Source: CAD feature listing. Evaluate the final solid. Frame: model axes, mm. A direction names the side the tool comes from. Give positions to 0.01 mm unless a question says otherwise; leave off trailing zeros. Order: outer loops, then holes, each group sorted by start corner. A loop starts at its lowest first (then second) coordinate and runs counter-clockwise, first axis right, second up.
```python
from build123d import *

# Parameters (mm, degrees)
SKETCH1_W           = 25.4
SKETCH1_H           = 23.622
BOSS_EXTRUDE1_DEPTH = 5.842
SKETCH2_R           = 3.175
CUT_EXTRUDE1_DEPTH  = 36.175102672
SKETCH3_R           = 7.14375
CUT_EXTRUDE2_DEPTH  = 4.9022
CUT_EXTRUDE3_DEPTH  = 36.175102672
CUT_EXTRUDE4_DEPTH  = 36.175102672
SKETCH6_W           = 7
SKETCH6_H           = 5
CUT_EXTRUDE5_DEPTH  = 36.175102828
SKETCH8_R           = 1.1303
CUT_EXTRUDE6_DEPTH  = 6.35


with BuildPart() as part:
    # Sketch1 → Boss-Extrude1 (new body)
    with BuildSketch(Plane(origin=(0, 0, 0), x_dir=(1, 0, 0), z_dir=(0, 1, 0))):
        with Locations((12.7, 11.811)):
            Rectangle(SKETCH1_W, SKETCH1_H)
    extrude(amount=BOSS_EXTRUDE1_DEPTH)

    # Sketch2 → Cut-Extrude1 (cut, through all)
    with BuildSketch(Plane(origin=(0, 5.842, 0), x_dir=(1, 0, 0), z_dir=(0, 1, 0))):
        with Locations(Location((12.7, 15.24, 0), (0, 0, 270))):
            Circle(SKETCH2_R)
    extrude(amount=-CUT_EXTRUDE1_DEPTH, mode=Mode.SUBTRACT)

    # Sketch3 → Cut-Extrude2 (cut)
    with BuildSketch(Plane(origin=(0, 5.842, 0), x_dir=(1, 0, 0), z_dir=(0, 1, 0))):
        with Locations(Location((12.7, 15.24, 0), (0, 0, 270))):
            Circle(SKETCH3_R)
    extrude(amount=-CUT_EXTRUDE2_DEPTH, mode=Mode.SUBTRACT)

    # Sketch4 → Cut-Extrude3 (cut, through all)
    with BuildSketch(Plane(origin=(0, 5.842, 0), x_dir=(1, 0, 0), z_dir=(0, 1, 0))):
        with BuildLine():
            ThreePointArc((4.318, 15.24), (6.77303096, 21.16696904), (12.7, 23.622))
            Line((12.7, 23.622), (0, 23.622))
            Line((0, 23.622), (0, 3.302))
            ThreePointArc((0, 3.302), (3.053287081, 4.566712919), (4.318, 7.62))
            Line((4.318, 7.62), (4.318, 15.24))
        make_face()
        with BuildLine():
            ThreePointArc((12.7, 23.622), (18.62696904, 21.16696904), (21.082, 15.24))
            Line((21.082, 15.24), (21.082, 7.62))
            ThreePointArc((21.082, 7.62), (22.346712919, 4.566712919), (25.4, 3.302))
            Line((25.4, 3.302), (25.4, 23.622))
            Line((25.4, 23.622), (12.7, 23.622))
        make_face()
    extrude(amount=-CUT_EXTRUDE3_DEPTH, mode=Mode.SUBTRACT)

    # Sketch5 → Cut-Extrude4 (cut, through all)
    with BuildSketch(Plane.XY):
        with BuildLine():
            Line((0, 0.920917387), (0, 0))
            Line((0, 0), (11.811, 0))
            ThreePointArc((11.811, 0), (5.887575951, 0.230578207), (0, 0.920917387))
        make_face()
        with BuildLine():
            ThreePointArc((25.4, 1.221475881), (18.632893512, 0.305983313), (11.811, 0))
            Line((11.811, 0), (25.4, 0))
            Line((25.4, 0), (25.4, 1.221475881))
        make_face()
    extrude(amount=-CUT_EXTRUDE4_DEPTH, mode=Mode.SUBTRACT)

    # Sketch6 → Cut-Extrude5 (cut, through all)
    with BuildSketch(Plane(origin=(0, 5.842, 0), x_dir=(1, 0, 0), z_dir=(0, 1, 0))):
        with Locations((12.700000015, 2.5)):
            Rectangle(SKETCH6_W, SKETCH6_H)
    extrude(amount=-CUT_EXTRUDE5_DEPTH, mode=Mode.SUBTRACT)

    # Sketch8 → Cut-Extrude6 (cut)
    with BuildSketch(Plane.XY):
        with Locations((5.390000015, 3.302)):
            Circle(SKETCH8_R)
        with Locations(Location((19.925856856, 3.487249582, 0), (0, 0, 180))):
            Circle(SKETCH8_R)
    extrude(amount=-CUT_EXTRUDE6_DEPTH, mode=Mode.SUBTRACT)


solid = part.part
```
1) Reachability of faces 1 (the flat face through (20, 3, -6.35)), 2 (the flat face through (16.2, 3, -2)), 3 (the flat face through (11, 0.94, -12)) from +Z, -Z, +X, -X, +Y, -Y: full face, straight path, thin tool, end or side. Return the list, or none.
Report:
face 1: +Z
face 2: +Z, +Y, -Y
face 3: +Y
2) Section query A-A, the plane x = 13.5. Return the cut outline in (y, z).
Report:
outline: (0.02, -23.58) - (5.84, -23.58) - (5.84, -22.34) - (0.94, -22.34) - (0.94, -18.31) - (0.02, -18.31) - close; (0.02, -12.17) - (0.94, -12.17) - (0.94, -8.14) - (5.84, -8.14) - (5.84, -5) - (0.02, -5) - close
3) Pin query (flat end, axial travel): pin 1 (1 mm diameter, centred on x = 4, z = -21, fed in from -Y); pin 2 (3 mm diameter, centred on x = 14.5, y = 2.5, fed in from -Z); pin 3 (1.8 mm diameter, centred on x = 20, y = 3.5, fed in from +Z); pin 4 (3.5 mm diameter, centred on x = 5.39, y = 3.302, fed in from -Z). Return the tip coordinate at first contact, or that it passes through.
Report:
pin 1: passes through
pin 2: stops at z = -23.62
pin 3: stops at z = -6.35
pin 4: stops at z = -21.51
4) Section query D-D, the plane x = 6. Return the cut outline in (y, z).
Report:
outline: (0.22, -20.28) - (5.84, -20.28) - (5.84, -17.72) - (0.94, -17.72) - (0.94, -12.76) - (5.84, -12.76) - (5.84, 0) - (4.25, 0) - (4.25, -6.35) - (2.35, -6.35) - (2.35, 0) - (0.22, 0) - close
5) Section query C-C, the plane z = -20. Return the cut outline in (x, y).
Report:
outline: (5.8, 0.24) arc R76.2 ccw to (19.6, 0.4) - (19.6, 5.84) - (18.03, 5.84) - (18.03, 0.94) - (7.37, 0.94) - (7.37, 5.84) - (5.8, 5.84) - close
6) Section query B-B, the plane y = 4.1. Return the cut outline in (x, z), and give its area (3 significant figures).
Report:
outline: (0, -3.3) arc R4.32 cw to (4.32, -7.62) - (4.32, -15.24) arc R8.38 ccw to (21.08, -15.24) - (21.08, -7.62) arc R4.32 cw to (25.4, -3.3) - (25.4, 0) - (20.88, 0) - (20.88, -6.35) - (18.98, -6.35) - (18.98, 0) - (16.2, 0) - (16.2, -5) - (9.2, -5) - (9.2, 0) - (6.19, 0) - (6.19, -6.35) - (4.59, -6.35) - (4.59, 0) - (0, 0) - close; hole circle Ø14.29 at (12.7, -15.24)
area: 185 mm2
7) Material intervals for L1, parallel to X at y = 0.7, z = -15.24 (3 decimals); L2, parallel to Y at x = 23.75, z = -2; L3, parallel to Z at x = 16, y = 2.05, sorted ascending.
Report:
L1: x = 4.318 to 9.525, 15.875 to 21.082
L2: y = 0.94 to 5.84
L3: z = -22.95 to -21.58, -8.9 to -5
8) Draft query along Y for faces 4 (the flat face through (5, 3, -6.35)), 5 (the flat face through (13, 5.842, -7)), 6 (the cylindrical face through (14.846, 3.425, -8.426)). Return one class per face: +Y half, -Y half, draft (parallel to the pull), parting line (faces both ways), or undercut.
Report:
face 4: undercut
face 5: +Y half
face 6: draft
